Design review of the part built by this model. Coordinates are the model's own, in mm. A direction names the side the tool comes from. Coordinates: 2 decimals unless noted, no trailing zeros. Order: outer loops, then holes, each group sorted by start corner. A loop starts at its lowest first (then second) coordinate and runs counter-clockwise, first axis right, second up.
from build123d import *

# Parameters (mm, degrees)
WYTNIJ_WYCI_GNI_CIE2_DEPTH = 4


with BuildPart() as part:
    # Szkic1 → Obrót1 (revolve)
    with BuildSketch(Plane.XY):
        Polygon((0, 0), (-50, 0), (-50, 3), (-4, 3), (-4, 7), (0, 7), align=None)
    revolve(axis=Axis((0, 0, 0), (-1, 0, 0)))

    # Szkic3 → Wytnij-wyciągnięcie2 (cut)
    with BuildSketch(Plane(origin=(0, 0, 0), x_dir=(0, 0, -1), z_dir=(1, 0, 0))):
        with BuildLine():
            Line((-7, 0), (-3.5, 6.062177826))
            ThreePointArc((-3.5, 6.062177826), (-6.062177826, 3.5), (-7, 0))
        make_face()
        with BuildLine():
            Line((-3.5, 6.062177826), (3.5, 6.062177826))
            ThreePointArc((3.5, 6.062177826), (0, 7), (-3.5, 6.062177826))
        make_face()
        with BuildLine():
            Line((3.5, 6.062177826), (7, 0))
            ThreePointArc((7, 0), (6.062177826, 3.5), (3.5, 6.062177826))
        make_face()
        with BuildLine():
            ThreePointArc((3.5, -6.062177826), (6.062177826, -3.5), (7, 0))
            Line((7, 0), (3.5, -6.062177826))
        make_face()
        with BuildLine():
            ThreePointArc((-3.5, -6.062177826), (0, -7), (3.5, -6.062177826))
            Line((3.5, -6.062177826), (-3.5, -6.062177826))
        make_face()
        with BuildLine():
            ThreePointArc((-7, 0), (-6.062177826, -3.5), (-3.5, -6.062177826))
            Line((-3.5, -6.062177826), (-7, 0))
        make_face()
    extrude(amount=-WYTNIJ_WYCI_GNI_CIE2_DEPTH, mode=Mode.SUBTRACT)


solid = part.part
1. Add section C-C (x = -40). Give the boundary of the cut face in (y, z), and give its area (3 significant figures).
2. Add section D-D (z = 4.75). Give the boundary of the cut face in (x, y), and give its area (3 significant figures).
3. To check wall thickness, follow line 1 (Y direction, x = -34.5, z = 0); line 2 (X direction, y = -1.75, z = -2.5); line 3 (Z direction, x = -29, y = 1). State the ranges of each line that lie inside material, in increasing order.
4. Insertion check: pin 1 (1.5 mm diameter, centred on y = 1, z = 3.5, fed in from -X); pin 2 (5 mm diameter, centred on x = -31.5, z = 3, fed in from -Y); pin 3 (8 mm diameter, centred on x = -24.5, z = -4, fed in from +Y); pin 4 (1.5 mm diameter, centred on x = -23, y = -2, fed in from +Z). Each pin has a flat end and moves straight along its axis. Give the tip position at first contact, or say it passes through.
5. For faces 1 (the flat face through (-4, 3, 1)), 2 (the flat face through (-2, 6.062, 0)), list the 3-axis set-ups (+Z, -Z, +X, -X, +Y, -Y) from which the entire face can be reached by the end or side of a thin tool; tool diameter is ignored.
6. Add section A-A (z = 0). Give the boundary of the cut face in (x, y), and give its area (3 significant figures).
7. Add section B-B (y = -2.5). Give the boundary of the cut face in (x, z), and give its area (3 significant figures).
Solution:
1. outline: circle Ø6 at (0, 0)
1. area: 28.3 mm2
2. outline: (-4, -3.9) - (0, -3.9) - (0, 3.9) - (-4, 3.9) - close
2. area: 31.2 mm2
3. line 1: y = -3 to 3
3. line 2: x = -4 to 0
3. line 3: z = -2.83 to 2.83
4. pin 1: stops at x = -50
4. pin 2: stops at y = -2.96
4. pin 3: stops at y = 3
4. pin 4: stops at z = 2.73
5. face 1: -X
5. face 2: +Z, -Z, +X, -X, +Y
6. outline: (-50, -3) - (-4, -3) - (-4, -6.06) - (0, -6.06) - (0, 6.06) - (-4, 6.06) - (-4, 3) - (-50, 3) - close
6. area: 324 mm2
7. outline: (-50, -1.66) - (-4, -1.66) - (-4, -5.56) - (0, -5.56) - (0, 5.56) - (-4, 5.56) - (-4, 1.66) - (-50, 1.66) - close
7. area: 197 mm2
